```python
from build123d import *

# Parameters (mm, degrees)
F0_R          = 38.1
F0_R_2        = 11.1125
F1_DEPTH      = 3.175
F1_DEPTH_BACK = 3.175
F3_DEPTH      = 25.4
F5_DEPTH      = 25.4
F6_T1_DEPTH   = 34.5170750052
F6_T3_DEPTH   = 35.0734141938
F6_T5_DEPTH   = 34.5549539208
F6_T7_DEPTH   = 35.3294952256
F6_T9_DEPTH   = 35.0734141938
F6_T11_DEPTH  = 34.5170750052
F6_T14_ANGLE  = 120.7671426779
F6_T16_ANGLE  = 119.4565466951
F6_T18_ANGLE  = 120.7671426779
F6_T22_ANGLE  = 120.7671426779
F6_T24_ANGLE  = 119.4565466951
F6_T26_ANGLE  = 120.7671426779


# Not quite as in the source:
# - a fillet or chamfer that OpenCascade refuses, or shapes differently, is made with other operations: its cross-section is extruded or revolved along the edge and cut away or added


with BuildPart() as f1:
    # F0 (on Top) → F1 (new body, two sides)
    with BuildSketch(Plane.XY) as f1_sk:
        Circle(F0_R)
        Circle(F0_R_2, mode=Mode.SUBTRACT)
    extrude(amount=F1_DEPTH)
    extrude(f1_sk.sketch, amount=-F1_DEPTH_BACK)

    # F2 (on face) → F3 (cut)
    with BuildSketch(Plane.XY.offset(3.175)):
        with BuildLine():
            Line((-32.9882322762, -19.0627), (0, 38.1))
            ThreePointArc((0, 38.1), (-32.9992338547, 19.0436489413), (-32.9882322762, -19.0627))
        make_face()
        with BuildLine():
            Line((32.9882322762, -19.0627), (-32.9882322762, -19.0627))
            ThreePointArc((-32.9882322762, -19.0627), (0, -38.1), (32.9882322762, -19.0627))
        make_face()
        with BuildLine():
            ThreePointArc((38.1, 0), (26.9407683632, 26.9407683632), (0, 38.1))
            Line((0, 38.1), (32.9882322762, -19.0627))
            ThreePointArc((32.9882322762, -19.0627), (36.7998753376, -9.8680887277), (38.1, 0))
        make_face()
    extrude(amount=-F3_DEPTH, mode=Mode.SUBTRACT)

    # F4 (on face) → F5 (cut)
    with BuildSketch(Plane.XY.offset(3.175)):
        with BuildLine():
            Line((-10.7228866295, 19.5191574013), (-21.9872687911, 0))
            ThreePointArc((-21.9872687911, 0), (-12.8675975863, 7.7469760001), (-10.7228866295, 19.5191574013))
        make_face()
        with BuildLine():
            Line((21.9872687911, 0), (10.7228866295, 19.5191574013))
            ThreePointArc((10.7228866295, 19.5191574013), (12.8675975863, 7.7469760001), (21.9872687911, 0))
        make_face()
        with BuildLine():
            ThreePointArc((11.4974279343, -19.0627), (0.3872706524, -15.1640834027), (-10.7228866295, -19.0627))
            Line((-10.7228866295, -19.0627), (11.4974279343, -19.0627))
        make_face()
    extrude(amount=-F5_DEPTH, mode=Mode.SUBTRACT)

    # F6: chamfer of 2.54 on 20 edges, made by hand

    # F6_s2 → F6_t1 (cut)
    with BuildSketch(Plane(origin=(-19.7590646722, 34.2389212213, 0), x_dir=(0, 0, 1), z_dir=(0.4998333055, -0.8661216235, 0))):
        Polygon((3.175, -16.5036489413), (0.635, -19.0436489413), (3.175, -19.0436489413), align=None)
        Polygon((-3.175, -16.5036489413), (-0.635, -19.0436489413), (-3.175, -19.0436489413), align=None)
    extrude(amount=F6_T1_DEPTH, mode=Mode.SUBTRACT)

    # F6_s4 → F6_t3 (cut)
    with BuildSketch(Plane(origin=(2.2282041189, -3.8610787787, 0), x_dir=(0, 0, 1), z_dir=(0.4998333055, -0.8661216235, 0))):
        Polygon((3.175, -16.5036489413), (0.635, -19.0436489413), (3.175, -19.0436489413), align=None)
        Polygon((-3.175, -16.5036489413), (-0.635, -19.0436489413), (-3.175, -19.0436489413), align=None)
    extrude(amount=F6_T3_DEPTH, mode=Mode.SUBTRACT)

    # F6_s6 → F6_t5 (cut)
    with BuildSketch(Plane.YZ.offset(4.9653531448)):
        Polygon((-16.5227, 3.175), (-19.0627, 0.635), (-19.0627, 3.175), align=None)
        Polygon((-16.5227, -3.175), (-19.0627, -0.635), (-19.0627, -3.175), align=None)
    extrude(amount=F6_T5_DEPTH, mode=Mode.SUBTRACT)

    # F6_s8 → F6_t7 (cut)
    with BuildSketch(Plane.YZ.offset(-39.5203070657)):
        Polygon((-16.5227, 3.175), (-19.0627, 0.635), (-19.0627, 3.175), align=None)
        Polygon((-16.5227, -3.175), (-19.0627, -0.635), (-19.0627, -3.175), align=None)
    extrude(amount=F6_T7_DEPTH, mode=Mode.SUBTRACT)

    # F6_s10 → F6_t9 (cut)
    with BuildSketch(Plane(origin=(-19.7590646722, -34.2389212213, 0), x_dir=(0, 0, 1), z_dir=(0.4998333055, 0.8661216235, 0))):
        Polygon((0.635, -19.0436489413), (3.175, -16.5036489413), (3.175, -19.0436489413), align=None)
        Polygon((-0.635, -19.0436489413), (-3.175, -16.5036489413), (-3.175, -19.0436489413), align=None)
    extrude(amount=F6_T9_DEPTH, mode=Mode.SUBTRACT)

    # F6_s12 → F6_t11 (cut)
    with BuildSketch(Plane(origin=(2.5062809746, 4.3429361799, 0), x_dir=(0, 0, 1), z_dir=(0.4998333055, 0.8661216235, 0))):
        Polygon((3.175, -16.5036489413), (0.635, -19.0436489413), (3.175, -19.0436489413), align=None)
        Polygon((-3.175, -16.5036489413), (-0.635, -19.0436489413), (-3.175, -19.0436489413), align=None)
    extrude(amount=F6_T11_DEPTH, mode=Mode.SUBTRACT)

    # F6_s13 → F6_t14 (revolve, cut)
    with BuildSketch(Plane(origin=(14.4954043102, 24.71215529, 0), x_dir=(0, 0, 1), z_dir=(0.505952459, 0.8625613655, 0))):
        Polygon((3.175, -4.353790183), (0.635, -1.813790183), (3.175, -1.813790183), align=None)
    revolve(axis=Axis((28.2672400519, 16.6340121728, 3.175), (0, 0, 1)), revolution_arc=F6_T14_ANGLE, mode=Mode.SUBTRACT)

    # F6_s15 → F6_t16 (revolve, cut)
    with BuildSketch(Plane(origin=(14.4410953434, -24.7409917864, 0), x_dir=(0, 0, 1), z_dir=(0.5041015086, -0.8636444112, 0))):
        Polygon((3.175, -4.0473019905), (0.635, -1.5073019905), (3.175, -1.5073019905), align=None)
    revolve(axis=Axis((0.3872706524, -32.9440834027, 3.175), (0, 0, 1)), revolution_arc=F6_T16_ANGLE, mode=Mode.SUBTRACT)

    # F6_s17 → F6_t18 (revolve, cut)
    with BuildSketch(Plane(origin=(-28.374198152, 0.1844947944, 0), x_dir=(0, 0, 1), z_dir=(-0.9999788613, 0.0065020655, 0))):
        Polygon((3.175, -3.8701348937), (0.635, -1.3301348937), (3.175, -1.3301348937), align=None)
    revolve(axis=Axis((-28.2672400519, 16.6340121728, 3.175), (0, 0, 1)), revolution_arc=F6_T18_ANGLE, mode=Mode.SUBTRACT)

    # F6_s19 → F6_t20 (revolve, cut)
    with BuildSketch(Plane.XZ):
        Polygon((13.6525, 3.175), (11.1125, 0.635), (11.1125, 3.175), align=None)
    revolve(axis=Axis((0, 0, 3.175), (0, 0, 1)), mode=Mode.SUBTRACT)

    # F6_s21 → F6_t22 (revolve, cut)
    with BuildSketch(Plane(origin=(14.4954043102, 24.71215529, 0), x_dir=(0, 0, 1), z_dir=(0.505952459, 0.8625613655, 0))):
        Polygon((-3.175, -4.353790183), (-0.635, -1.813790183), (-3.175, -1.813790183), align=None)
    revolve(axis=Axis((28.2672400519, 16.6340121728, -3.175), (0, 0, 1)), revolution_arc=F6_T22_ANGLE, mode=Mode.SUBTRACT)

    # F6_s23 → F6_t24 (revolve, cut)
    with BuildSketch(Plane(origin=(14.4410953434, -24.7409917864, 0), x_dir=(0, 0, 1), z_dir=(0.5041015086, -0.8636444112, 0))):
        Polygon((-3.175, -4.0473019905), (-0.635, -1.5073019905), (-3.175, -1.5073019905), align=None)
    revolve(axis=Axis((0.3872706524, -32.9440834027, -3.175), (0, 0, 1)), revolution_arc=F6_T24_ANGLE, mode=Mode.SUBTRACT)

    # F6_s25 → F6_t26 (revolve, cut)
    with BuildSketch(Plane(origin=(-28.374198152, 0.1844947944, 0), x_dir=(0, 0, 1), z_dir=(-0.9999788613, 0.0065020655, 0))):
        Polygon((-0.635, -1.3301348937), (-3.175, -3.8701348937), (-3.175, -1.3301348937), align=None)
    revolve(axis=Axis((-28.2672400519, 16.6340121728, -3.175), (0, 0, 1)), revolution_arc=F6_T26_ANGLE, mode=Mode.SUBTRACT)

    # F6_s27 → F6_t28 (revolve, cut)
    with BuildSketch(Plane.XZ):
        Polygon((13.6525, -3.175), (11.1125, -0.635), (11.1125, -3.175), align=None)
    revolve(axis=Axis((0, 0, -3.175), (0, 0, 1)), mode=Mode.SUBTRACT)


solid = f1.part
```
Here's how the part is built. I have some questions about the finished solid (model axes, mm). Give positions to 0.01 mm unless a question says otherwise; leave off trailing zeros. Loops run counter-clockwise (first coordinate to the right, second up) from the corner with the lowest first, then second, coordinate; pieces in that order, holes last. Notation, with made-up numbers: (15, 6.25) -> (68, 6.25) arc R12 cw to (68, 18.25) -> close; hole circle Ø4 at (35.25, 3). An arc over 180 degrees is marked (long way). Use one line per item in the form item = value. Start each with the question number.
1) Please list where these lines run through material, in increasing order: line 1 along Y through (x, z) = (-7.5, 2.5); line 2 along X through (y, z) = (-7, -0.25); line 3 along Y through (x, z) = (1, 2.5).
2) For P1, Ø2, axis at x = -7.5, z = 1, coming from the +Y side; P2, Ø3, axis at y = 12.5, z = 1.5, coming from the -X side; P3, Ø1, axis at y = 23, z = 2.5, coming from the +X side, each with a flat end and sliding along its axis, tell me the tip position at first contact or that it passes through.
3) Imagine slicing it at B-B (y = 21). Please give me the cut outline in (x, z) (3 decimals), then the cut area to 3 significant figures.
4) Thinking about a two-plate mould opening in X: for faces 1 (the face through (-12.954, 7.599, 0.009)), 2 (the face through (0.6, -14.8, 1)), 3 (the face through (-22, -17.8, -1.9)), 4 (the face through (10.6, 3.34, -0.01)), which applies, +X half, -X half, draft (parallel to the pull), parting line (faces both ways), or undercut?
5) Imagine slicing it at C-C (x = 27). Please give me the cut outline in (y, z) (3 decimals), then the cut area to 3 significant figures.
6) Imagine slicing it at A-A (z = -1.75). Please give me the cut outline in (x, y) (1 decimal).
Check values:
q1.line_1 = -14.95 to -10.59, 10.59 to 21.37
q1.line_2 = -26.03 to -8.63, 8.63 to 26.03
q1.line_3 = -13.31 to -12.94, 12.94 to 32.64
q2.P1 = 26.72
q2.P2 = -11.31
q2.P3 = 7.21
q3.outline = (-9.868, -0.635) -> (-6.936, -3.175) -> (6.936, -3.175) -> (9.868, -0.635) -> (9.868, 0.635) -> (6.936, 3.175) -> (-6.936, 3.175) -> (-9.868, 0.635) -> close
q3.area = 110 mm^2
q4.face_1 = -X half
q4.face_2 = undercut
q4.face_3 = draft
q4.face_4 = undercut
q5.outline = (-19.063, -0.635) -> (-16.523, -3.175) -> (-13.768, -3.175) -> (-8.686, -0.635) -> (-8.686, 0.635) -> (-13.768, 3.175) -> (-16.523, 3.175) -> (-19.063, 0.635) -> close
q5.area = 46.5 mm^2
q6.outline = (-31.1, -17.9) -> (-11.1, -17.9) arc R18.9 cw to (11.9, -17.9) -> (31.1, -17.9) -> (21.2, -0.9) arc R18.9 cw to (9.6, 19.3) -> (0, 35.9) -> (-9.6, 19.3) arc R18.9 cw to (-21.2, -0.9) -> close; hole circle Ø24.5 at (0, 0)
